Read the model definition and answer for the solid it produces. Units are mm, in the model's axes. Face numbers are marked on the shaded views. A direction names the side the tool comes from. Coordinates: 2 decimals unless noted, no trailing zeros. Loops run counter-clockwise (first coordinate to the right, second up) from the corner with the lowest first, then second, coordinate; pieces in that order, holes last. Notation, with made-up numbers: (9, -22) -> (68, -22) arc R12 ccw to (68, -4) -> close; hole circle Ø1 at (-31, 84.5). An arc over 180 degrees is marked (long way). Answer as a JSON object with one key per item and string values. Group by question number.
Q1. For the marked faces 1, 2 and 3, determine the directions among +Z, -Z, +X, -X, +Y, -Y from which every point of the face is accessible in a straight line to the end or side of a thin tool.
Q2. Straight lines are drawn through the part: line 1 along X through (y, z) = (-4, 19); line 2 along Z through (x, y) = (29, -12). For each, find the intervals that lie inside material, in ascending order. Write a range as [from, to].
Q3. The part is cut by section A-A on z = 19.05. State how many separate pieces and enclosed holes the cut face has, and give its area (3 significant figures).
Q4. The part is cut by section C-C on y = -20.32. Write down the section's boundary in (x, z).
Q5. Each of these flat-tipped pins is pushed along its axis until it touches: P1, Ø7.5, axis at x = 15.63, z = 19.05, coming from the -Y side; P2, Ø16.5, axis at x = 22, y = -15, coming from the +Z side; P3, Ø5.5, axis at x = 47.625, y = -20.32, coming from the +Z side. Where does it stop, or does it pass through?
from build123d import *

# Parameters (mm, degrees)
F1_DEPTH = 5.08
F2_W     = 63.5
F2_H     = 6.35
F3_DEPTH = 25.4
F4_R     = 2.3114
F5_DEPTH = 25.4
F6_SIZE  = 5.07999


# Not quite as in the source:
# - a fillet or chamfer is up to 0.001 mm smaller than in the source, because OpenCascade refuses the exact size


with BuildPart() as f1:
    # F0 (on Front) → F1 (new body)
    with BuildSketch(Plane.XZ):
        Polygon((0, 19.05), (0, 0), (31.75, 0), (31.75, 38.1), (30.7521958955, 38.1), (0, 38.1), align=None)
        with BuildLine():
            ThreePointArc((17.9369489739, 19.05), (15.6255489739, 16.7386), (13.3141489739, 19.05))
            ThreePointArc((13.3141489739, 19.05), (15.6255489739, 21.3614), (17.9369489739, 19.05))
        make_face(mode=Mode.SUBTRACT)
        Polygon((31.75, 38.1), (31.75, 0), (63.5, 0), (63.5, 19.05), (63.5, 38.1), (32.7478041045, 38.1), align=None)
        with BuildLine():
            ThreePointArc((45.5630510261, 19.05), (47.8744510261, 21.3614), (50.1858510261, 19.05))
            ThreePointArc((50.1858510261, 19.05), (47.8744510261, 16.7386), (45.5630510261, 19.05))
        make_face(mode=Mode.SUBTRACT)
    extrude(amount=F1_DEPTH)

    # F2 (on face) → F3 (join)
    with BuildSketch(Plane.XZ.offset(5.08)):
        with Locations((31.75, 3.175)):
            Rectangle(F2_W, F2_H)
    extrude(amount=F3_DEPTH)

    # F4 (on face) → F5 (cut)
    with BuildSketch(Plane.XY.offset(6.35)):
        with Locations((15.875, -20.32)):
            Circle(F4_R)
        with Locations((47.625, -20.32)):
            Circle(F4_R)
    extrude(amount=-F5_DEPTH, mode=Mode.SUBTRACT)

    # F6 (size 5.08 in the source; OpenCascade refuses exactly that, so slightly less here)
    f6_edges = [f1.edges().sort_by_distance(p)[0] for p in [
        (31.75, -5.08, 38.1),
        (31.75, -30.48, 6.35),
        (0, -17.78, 6.35),
        (63.5, -17.78, 6.35),
        (0, -5.08, 22.225),
        (63.5, -5.08, 22.225),
    ]]
    chamfer(f6_edges, length=F6_SIZE)


solid = f1.part
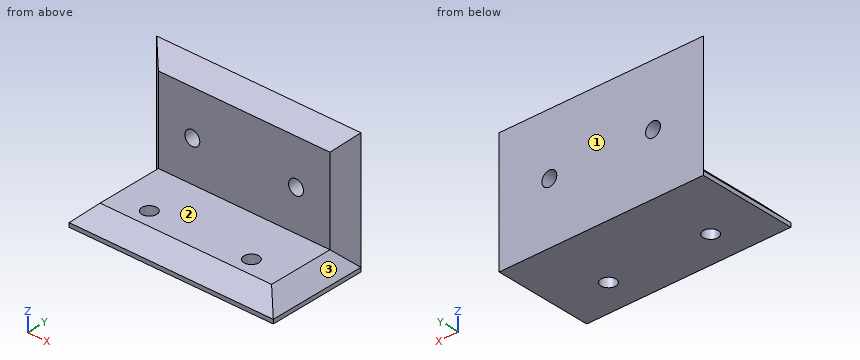
Final values:
{
 "1": {"face 1": "+Z, -Z, +X, -X, +Y", "face 2": "+Z, +X, -X, -Y", "face 3": "+Z, +X, -Y"},
 "2": {"line 1": "x = [4, 13.31], [17.94, 45.56], [50.19, 59.5]", "line 2": "z = [0, 6.35]"},
 "3": {"separate pieces": "3", "enclosed holes": "0", "area": "250 mm2"},
 "4": {"outline": "(0, 0) -> (13.56, 0) -> (13.56, 6.35) -> (5.08, 6.35) -> (0, 1.27) -> close; (18.19, 0) -> (45.31, 0) -> (45.31, 6.35) -> (18.19, 6.35) -> close; (49.94, 0) -> (63.5, 0) -> (63.5, 1.27) -> (58.42, 6.35) -> (49.94, 6.35) -> close"},
 "5": {"P1": "stops at y = -5.08", "P2": "stops at z = 6.35", "P3": "stops at z = 6.35"}
}
